from build123d import *

# Parameters (mm, degrees)
ESQUISSE1_R             = 13.85
BOSS_EXTRU_1_DEPTH      = 32.5
ESQUISSE1_3_R           = 5
BOSS_EXTRU_2_DEPTH      = 36
BOSS_EXTRU_2_DEPTH_BACK = 2.2
ESQUISSE1_4_R           = 1.1525
BOSS_EXTRU_3_DEPTH      = 44
BOSS_EXTRU_3_DEPTH_BACK = 3
ESQUISSE1_5_W           = 0.4
ESQUISSE1_5_H           = 2.8
BOSS_EXTRU_4_DEPTH      = 5.5
ENL_V_MAT_EXTRU_2_REACH = 24.25
ESQUISSE2_RX            = 1.263747853
ESQUISSE2_RY            = 0.805399752
ENL_V_MAT_EXTRU_3_REACH = 24.25
ESQUISSE3_RX            = 1.263747853
ESQUISSE3_RY            = 0.805399752


with BuildPart() as part:
    # Esquisse1 → Boss.-Extru.1 (new body)
    with BuildSketch(Plane(origin=(0, 0, 0), x_dir=(1, 0, 0), z_dir=(0, 1, 0))):
        Circle(ESQUISSE1_R)
    extrude(amount=BOSS_EXTRU_1_DEPTH)

    # Esquisse1_3 → Boss.-Extru.2 (add, two sides)
    with BuildSketch(Plane(origin=(0, 0, 0), x_dir=(1, 0, 0), z_dir=(0, 1, 0))) as boss_extru_2_sk:
        Circle(ESQUISSE1_3_R)
    extrude(amount=BOSS_EXTRU_2_DEPTH)
    extrude(boss_extru_2_sk.sketch, amount=-BOSS_EXTRU_2_DEPTH_BACK)

    # Esquisse1_4 → Boss.-Extru.3 (add, two sides)
    with BuildSketch(Plane(origin=(0, 0, 0), x_dir=(1, 0, 0), z_dir=(0, 1, 0))) as boss_extru_3_sk:
        Circle(ESQUISSE1_4_R)
    extrude(amount=BOSS_EXTRU_3_DEPTH)
    extrude(boss_extru_3_sk.sketch, amount=-BOSS_EXTRU_3_DEPTH_BACK)

    # Esquisse1_5 → Boss.-Extru.4 (add)
    with BuildSketch(Plane(origin=(0, 0, 0), x_dir=(1, 0, 0), z_dir=(0, 1, 0))):
        with Locations((-8.2, 0)):
            Rectangle(ESQUISSE1_5_W, ESQUISSE1_5_H)
        with Locations((8.2, 0)):
            Rectangle(ESQUISSE1_5_W, ESQUISSE1_5_H)
    extrude(amount=-BOSS_EXTRU_4_DEPTH)

    # Esquisse2 → Enl_v. mat.-Extru.2 (cut, up to next)
    with BuildSketch(Plane.ZY.offset(8.4), mode=Mode.PRIVATE) as enl_v_mat_extru_2_sk1:
        with Locations(Location((0, -3.697573844), (0, 0, 90))):
            Ellipse(ESQUISSE2_RX, ESQUISSE2_RY)
    enl_v_mat_extru_2_tool1 = extrude(enl_v_mat_extru_2_sk1.sketch, amount=-ENL_V_MAT_EXTRU_2_REACH, mode=Mode.PRIVATE) & part.part
    add(enl_v_mat_extru_2_tool1.solids().sort_by_distance((-8.4, -3.697574, 0))[0], mode=Mode.SUBTRACT)

    # Esquisse3 → Enl_v. mat.-Extru.3 (cut, up to next)
    with BuildSketch(Plane(origin=(8.4, 0, 0), x_dir=(0, 0, -1), z_dir=(1, 0, 0)), mode=Mode.PRIVATE) as enl_v_mat_extru_3_sk1:
        with Locations(Location((0, -3.697573844), (0, 0, -90))):
            Ellipse(ESQUISSE3_RX, ESQUISSE3_RY)
    enl_v_mat_extru_3_tool1 = extrude(enl_v_mat_extru_3_sk1.sketch, amount=-ENL_V_MAT_EXTRU_3_REACH, mode=Mode.PRIVATE) & part.part
    add(enl_v_mat_extru_3_tool1.solids().sort_by_distance((8.4, -3.697574, 0))[0], mode=Mode.SUBTRACT)


solid = part.part
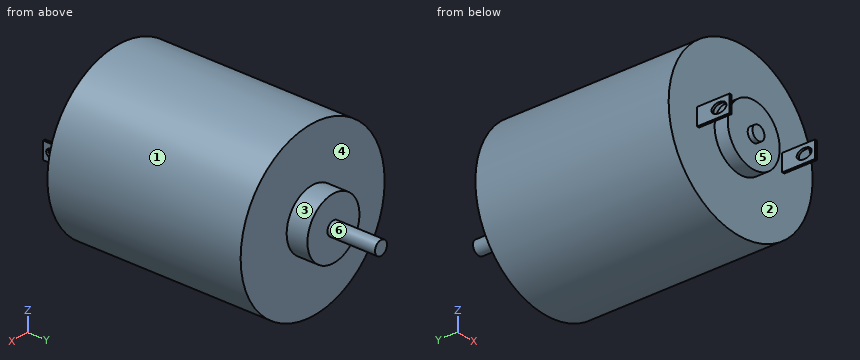
The model under review builds one solid part; all positions refer to its coordinate system, in mm. Face numbers are marked on the shaded views. A direction names the side the tool comes from. Coordinates: 2 decimals unless noted, no trailing zeros. Write each loop counter-clockwise with the first axis right and the second up, starting at its lowest first coordinate (ties: lowest second). Pieces come first, ordered by that corner, then holes. Notation, with made-up numbers: (13, -36.5) - (54, -36.5) arc R18 ccw to (54, -17.5) - close; hole circle Ø5 at (-17, 89). An arc over 180 degrees is marked (long way). Answer as CSV lines item,"result".
(1) Clearance check with flat-ended pins moving along their axes: pin 1 Ø2 at (x, z) = (9.5, 2.5) entering from -Y; pin 2 Ø10 at (x, z) = (7, 6.5) entering from +Y; pin 3 Ø1 at (y, z) = (10, 2) entering from -X; pin 4 Ø0.8 at (y, z) = (-4, 0) entering from -X. State where each tip first meets the part, or that it passes through.
Data:
pin 1,"stops at y = 0"
pin 2,"stops at y = 36"
pin 3,"stops at x = -13.77"
pin 4,"passes through"
(2) We need section C-C (y = 19). Give the boundary of the cut face in (x, z).
Data:
outline,"circle Ø27.7 at (0, 0)"
(3) We need section A-A (z = 0). Count the separate pieces of the cut face and the enclosed holes in it, plus the area to 3 significant figures.
Data:
separate pieces,"3"
enclosed holes,"0"
area,"980 mm2"
(4) We need section D-D (z = 4.25). Give the boundary of the cut face in (x, y), plus the area to 3 significant figures.
Data:
outline,"(-13.18, 0) - (-2.63, 0) - (-2.63, -2.2) - (2.63, -2.2) - (2.63, 0) - (13.18, 0) - (13.18, 32.5) - (2.63, 32.5) - (2.63, 36) - (-2.63, 36) - (-2.63, 32.5) - (-13.18, 32.5) - close"
area,"887 mm2"
(5) We need section B-B (x = 0). Give the boundary of the cut face in (y, z).
Data:
outline,"(-3, -1.15) - (-2.2, -1.15) - (-2.2, -5) - (0, -5) - (0, -13.85) - (32.5, -13.85) - (32.5, -5) - (36, -5) - (36, -1.15) - (44, -1.15) - (44, 1.15) - (36, 1.15) - (36, 5) - (32.5, 5) - (32.5, 13.85) - (0, 13.85) - (0, 5) - (-2.2, 5) - (-2.2, 1.15) - (-3, 1.15) - close"
(6) Tool access review of the marked faces 1, 2 and 3: name each direction out of +Z, -Z, +X, -X, +Y, -Y from which nothing blocks a thin tool from reaching the whole face with its end or side.
Data:
face 1,"+Y, -Y"
face 2,"-Y"
face 3,"+Y"
(7) For line 1 along Y through (x, z) = (5.5, -9.75); line 2 along Y through (x, z) = (1, -4); line 3 along Z through (x, y) = (1.5, 8), list the stretches that pass through material, from the lowest coordinate up. Write a range as [from, to].
Data:
line 1,"y = [0, 32.5]"
line 2,"y = [-2.2, 36]"
line 3,"z = [-13.77, 13.77]"
(8) Mouldability with a two-part tool opening along X and no side actions: class the marked faces 4, 5 and 6 as pulls with the +X half, pulls with the -X half, needs draft (parallel to the pull), parting line crosses it, or undercut.
Data:
face 4,"needs draft"
face 5,"undercut"
face 6,"parting line crosses it"
